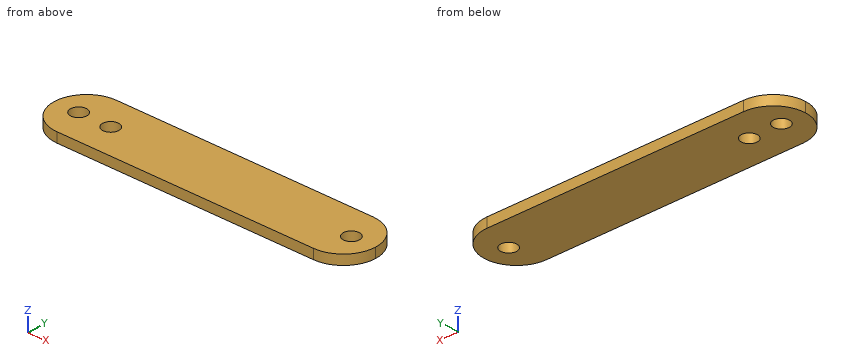
Autodesk Inventor part; units mm, degrees
ref_plane "YZ Plane" through (0, 0, 0) normal (1, 0, 0) x (0, 1, 0)
ref_plane "XZ Plane" through (0, 0, 0) normal (0, 1, 0) x (-1, 0, 0)
ref_plane "XY Plane" through (0, 0, 0) normal (0, 0, 1) x (1, 0, 0)
sketch "Sketch1" plane through (0, 0, 0) normal (0, 0, 1) x (1, 0, 0)
  line L0 (0, 0) -> (0, -20)
  line L1 (0, -20) -> (100, -20)
  line L2 (100, -20) -> (100, 0)
  line L3 (100, 0) -> (0, 0)
  line L4 (0, 0) -> (0, -10)
  line L5 (0, -10) -> (7.5, -10)
  circle A0 centre (7.5, -10) radius 2.5
  circle A1 centre (92.5, -10) radius 2.5
  dimension "d2" = 10
  dimension "d3" = 7.5
  dimension "d4" = 5
  dimension "d5" = 5
  dimension "d6" = 7.5
extrude "Extrusion1" add sketch "Sketch1" along normal blind 3
fillet "Fillet1" radius 10 1 edges at (100, 0, 1.5)
fillet "Fillet2" radius 10 1 edges at (100, -20, 1.5)
fillet "Fillet3" radius 10 1 edges at (0, -20, 1.5)
fillet "Fillet4" radius 10 1 edges at (0, 0, 1.5)
sketch "Sketch2" plane through (0, 0, 0) normal (0, 0, -1) x (-1, 0, 0)
  circle A0 centre (-7.5, -10) radius 2.5
  circle A1 centre (-17.5, -10) radius 2.5
  point P0 (0, 0)
extrude "Extrusion2" cut sketch "Sketch2" against normal through all contours A1
properties part number "new acr connect" material "Glass"
The listing builds one solid part. Answer for the finished solid, in the listing's coordinates (mm). Give positions to 0.01 mm unless a question says otherwise; leave off trailing zeros. Write each loop counter-clockwise with the first axis right and the second up, starting at its lowest first coordinate (ties: lowest second). Pieces come first, ordered by that corner, then holes.
Item 1: Find the intervals of material crossed by line 1 along X through (y, z) = (-11.5, 0.6); line 2 along Y through (x, z) = (17.5, 2); line 3 along X through (y, z) = (-9.25, 1.1), in increasing order.
Item 2: Section A-A, the plane x = 17.5 is taken. Write down the section's boundary in (y, z).
Item 3: Section C-C, the plane y = -1.75 is taken. Write down the section's boundary in (x, z), plus the area to 3 significant figures.
Item 4: Section D-D, the plane y = -5.5 is taken. Write down the section's boundary in (x, z).
Item 5: Section B-B, the plane x = 92.5 is taken. Write down the section's boundary in (y, z), plus the area to 3 significant figures.
Item 6: Flat-ended cylindrical pins translate along their axes: P1, Ø6, axis at x = 7.5, y = -10, coming from the -Z side; P2, Ø1, axis at y = -15.5, z = 2.5, coming from the +X side. Find the tip coordinate at first contact, or state that the pin passes through.
Completed:
1. line 1: x = 0.11 to 5.5, 9.5 to 15.5, 19.5 to 90.5, 94.5 to 99.89
1. line 2: y = -20 to -12.5, -7.5 to 0
1. line 3: x = 0.03 to 5.12, 9.88 to 15.12, 19.88 to 90.12, 94.88 to 99.97
2. outline: (-20, 0) - (-12.5, 0) - (-12.5, 3) - (-20, 3) - close; (-7.5, 0) - (0, 0) - (0, 3) - (-7.5, 3) - close
3. outline: (4.35, 0) - (95.65, 0) - (95.65, 3) - (4.35, 3) - close
3. area: 274 mm2
4. outline: (1.07, 0) - (98.93, 0) - (98.93, 3) - (1.07, 3) - close
5. outline: (-19.68, 0) - (-12.5, 0) - (-12.5, 3) - (-19.68, 3) - close; (-7.5, 0) - (-0.32, 0) - (-0.32, 3) - (-7.5, 3) - close
5. area: 43.1 mm2
6. P1: stops at z = 0
6. P2: stops at x = 98.66
